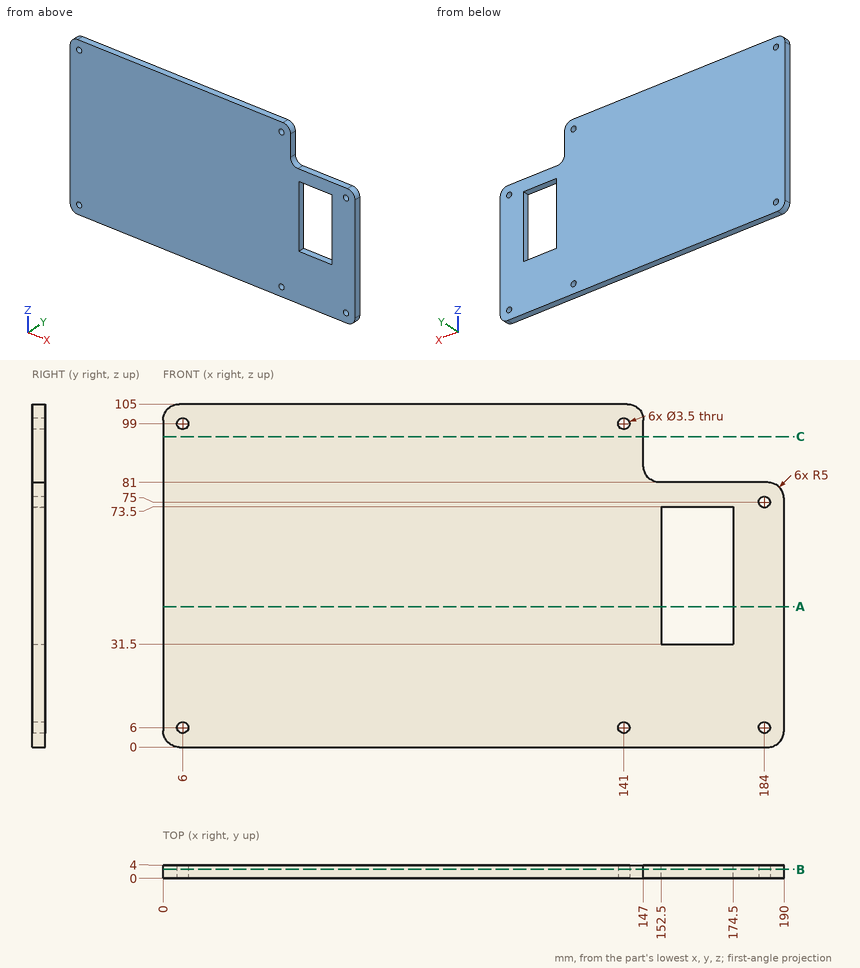
Drawing for the job (mm, zero at the part's lowest x, y, z). Coordinates: 2 decimals unless noted, no trailing zeros. Write each loop counter-clockwise with the first axis right and the second up, starting at its lowest first coordinate (ties: lowest second). Pieces come first, ordered by that corner, then holes. Notation, with made-up numbers: (78, 40.5) -> (83, 40.5) arc R15 ccw to (83, 67.5) -> close; hole circle Ø4 at (-13, 25). An arc over 180 degrees is marked (long way). One line per item, written item: value. Start each with the question number.
1) Slice it at C-C on z = 95. Write the cut outline in (x, y).
2) Slice it at A-A on z = 43. Write the cut outline in (x, y).
3) Slice it at B-B on y = 2.7. Write the cut outline in (x, z), then the cut area to 3 significant figures.
4) Probe probe 1 along X at (y, z) = (2.95, 99); probe 2 along X at (y, z) = (1.9, 6); probe 3 along X at (y, z) = (1.05, 75). List the from-to ranges inside material, lowest first.
5) Flat gauge pins, fed straight in: pin 1 Ø4 at (x, z) = (141, 99) entering from +Y; pin 2 Ø2 at (x, y) = (159.5, 2) entering from +Z. Where does each tip first touch, or does it go through?
Answers follow:
1. outline: (0, 0) -> (147, 0) -> (147, 4) -> (0, 4) -> close
2. outline: (0, 0) -> (152.5, 0) -> (152.5, 4) -> (0, 4) -> close; (174.5, 0) -> (190, 0) -> (190, 4) -> (174.5, 4) -> close
3. outline: (0, 5) arc R5 ccw to (5, 0) -> (185, 0) arc R5 ccw to (190, 5) -> (190, 76) arc R5 ccw to (185, 81) -> (152, 81) arc R5 cw to (147, 86) -> (147, 100) arc R5 ccw to (142, 105) -> (5, 105) arc R5 ccw to (0, 100) -> close; hole circle Ø3.5 at (6, 6); hole circle Ø3.5 at (6, 99); hole circle Ø3.5 at (141, 6); hole circle Ø3.5 at (141, 99); hole (152.5, 31.5) -> (174.5, 31.5) -> (174.5, 73.5) -> (152.5, 73.5) -> close; hole circle Ø3.5 at (184, 6); hole circle Ø3.5 at (184, 75)
3. area: 17,900 mm2
4. probe 1: 0 to 4.25, 7.75 to 139.25, 142.75 to 147
4. probe 2: 0 to 4.25, 7.75 to 139.25, 142.75 to 182.25, 185.75 to 190
4. probe 3: 0 to 182.25, 185.75 to 190
5. pin 1: y = 4
5. pin 2: z = 81
